Geometry: final body of the model. Coordinates: model frame, mm. Face numbers are marked on the shaded views. A direction names the side the tool comes from. Give positions to 0.01 mm unless a question says otherwise; leave off trailing zeros. Write each loop counter-clockwise with the first axis right and the second up, starting at its lowest first coordinate (ties: lowest second). Pieces come first, ordered by that corner, then holes. Notation, with made-up numbers: (68.25, 68.5) -> (82.25, 68.5) arc R20 cw to (82.25, 97.5) -> close; hole circle Ø11 at (58, 32). An arc over 180 degrees is marked (long way). Use CSV: the item, a comma, the result in double quotes. Start each with the question number.
1) Set-up query: the marked faces 1 and 2. Return all of +Z, -Z, +X, -X, +Y, -Y with unobstructed straight access to the full face (end or side cutting, diameter ignored); none if empty.
2) Section B-B (y = 13). Output: boundary loops of the cut face in (x, z).
3) Material intervals for line 1 (X direction, y = 14, z = 1); line 2 (X direction, y = 1.75, z = 4); line 3 (X direction, y = 0.25, z = 7.75), sorted ascending. Write a range as [from, to].
4) Section A-A (z = 7). Output: boundary loops of the cut face in (x, y).
5) Section C-C (x = 23). Output: boundary loops of the cut face in (y, z).
6) Draft query along X for the marked faces 3, 4, 5 and 6. Return one class per face: pulls with the +X half, pulls with the -X half, needs draft (parallel to the pull), parting line crosses it, or undercut.
Autodesk Fusion 360 part; units mm, degrees
sketch "Schizzo1" plane through (0, 0, 0) normal (0, 0, 1) x (1, 0, 0)
  line L0 (-35.7529, 16.0578) -> (-5.7529, 16.0578)
  line L1 (-5.7529, 16.0578) -> (-5.7529, -13.9422)
  line L2 (-5.7529, -13.9422) -> (-35.7529, -13.9422)
  line L3 (-35.7529, -13.9422) -> (-35.7529, 16.0578)
  line L4 (-5.7529, 16.0578) -> (44.2471, 16.0578)
  line L5 (44.2471, 16.0578) -> (44.2471, -13.9422)
  line L6 (44.2471, -13.9422) -> (-5.7529, -13.9422)
  line L7 (36.2471, 16.0578) -> (36.2471, -13.9422) construction
  line L8 (44.2471, 1.0578) -> (-5.7529, 1.0578) construction
  circle A0 centre (36.2471, 1.0578) radius 2.5
  line L9 (28.2471, 16.0578) -> (28.2471, -13.9422)
  line L10 (6.9284, 1.1522) -> (17.2791, 1.0578) construction
  line L11 (17.2791, 1.0578) -> (17.3507, 8.9056) construction
  line L12 (17.3507, 8.9056) -> (7, 9) construction
  line L13 (7, 9) -> (6.9284, 1.1522) construction
  dimension "d1" = 30
  dimension "d2" = 30
  dimension "d3" = 50
  dimension "d4" = 30
  dimension "d5" = 8
  dimension "d6" = 5
  dimension "d13" = 8
  dimension "d14" = 10
  dimension "d15" = 0
  dimension "d21" = 80
extrude "Estrusione1" add sketch "Schizzo1" along normal blind 10 contours L0 L1 L2 L3
extrude "Estrusione2" add sketch "Schizzo1" along normal blind 0.6 contours L1 L4 L6 L9
extrude "Estrusione3" add sketch "Schizzo1" along normal up to surface (10 mm away) contours L4 L5 L6 L9
extrude "Estrusione4" [suppressed]
extrude "Estrusione5" [suppressed]
equation "d13 = d5"
equation "d15 = '10.0'"
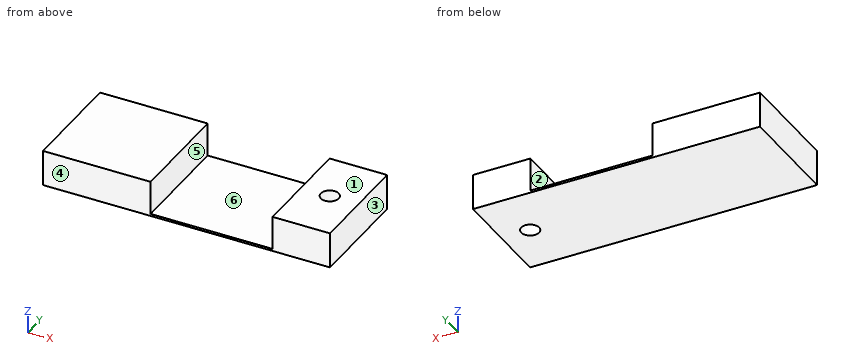
Answers follow:
1,face 1,"+Z, +X, -X, +Y, -Y"
1,face 2,"+Z, +Y, -Y"
2,outline,"(-35.75, 0) -> (44.25, 0) -> (44.25, 10) -> (28.25, 10) -> (28.25, 0.6) -> (-5.75, 0.6) -> (-5.75, 10) -> (-35.75, 10) -> close"
3,line 1,"x = [-35.75, -5.75], [28.25, 44.25]"
3,line 2,"x = [-35.75, -5.75], [28.25, 33.84], [38.65, 44.25]"
3,line 3,"x = [-35.75, -5.75], [28.25, 33.88], [38.61, 44.25]"
4,outline,"(-35.75, -13.94) -> (-5.75, -13.94) -> (-5.75, 16.06) -> (-35.75, 16.06) -> close; (28.25, -13.94) -> (44.25, -13.94) -> (44.25, 16.06) -> (28.25, 16.06) -> close; hole circle Ø5 at (36.25, 1.06)"
5,outline,"(-13.94, 0) -> (16.06, 0) -> (16.06, 0.6) -> (-13.94, 0.6) -> close"
6,face 3,"pulls with the +X half"
6,face 4,"needs draft"
6,face 5,"undercut"
6,face 6,"undercut"
